Geometry: final body of the model. Coordinates: model frame, mm. Face numbers are marked on the shaded views. A direction names the side the tool comes from. Round coordinates to 2 decimals unless told otherwise and drop trailing zeros. Write each loop counter-clockwise with the first axis right and the second up, starting at its lowest first coordinate (ties: lowest second). Pieces come first, ordered by that corner, then holes. Notation, with made-up numbers: M 48,-34 L 74,-34 A20 cw 74,1 Z; hole C 14.5,78.5 d10. An arc over 180 degrees is marked long. Use one line per item in the form item = value. Start each with the question number.
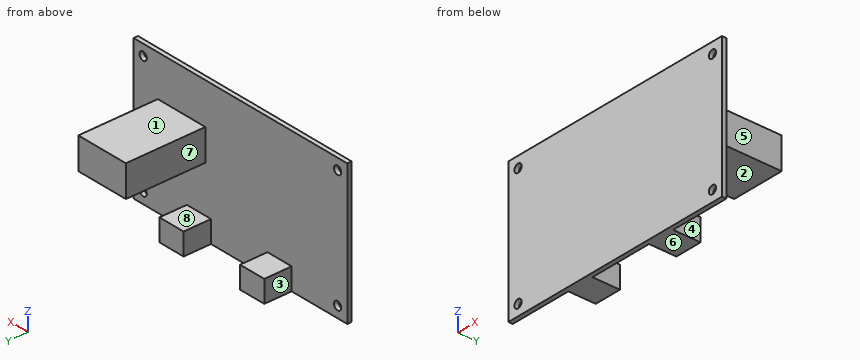
from build123d import *

# Parameters (mm, degrees)
ESQUISSE1_W        = 88.36
ESQUISSE1_H        = 51.38
ESQUISSE1_R        = 1.5
BOSS_EXTRU_2_DEPTH = 1.6
ESQUISSE3_W        = 10
ESQUISSE3_H        = 8
BOSS_EXTRU_3_DEPTH = 10
ESQUISSE4_W        = 19.65008467
ESQUISSE4_H        = 11.451158756
BOSS_EXTRU_4_DEPTH = 29


with BuildPart() as part:
    # Esquisse1 → Boss.-Extru.2 (new body)
    with BuildSketch(Plane(origin=(0, 0, 0), x_dir=(1, 0, 0), z_dir=(0, 1, 0))):
        with Locations((12.941904762, 5.88047619)):
            Rectangle(ESQUISSE1_W, ESQUISSE1_H)
        with Locations(Location((-27.238095238, -15.80952381, 0), (0, 0, 270))):
            Circle(ESQUISSE1_R, mode=Mode.SUBTRACT)
        with Locations(Location((53.171904762, -15.80952381, 0), (0, 0, 270))):
            Circle(ESQUISSE1_R, mode=Mode.SUBTRACT)
        with Locations(Location((53.171904762, 27.55047619, 0), (0, 0, 270))):
            Circle(ESQUISSE1_R, mode=Mode.SUBTRACT)
        with Locations(Location((-27.238095238, 27.55047619, 0), (0, 0, 270))):
            Circle(ESQUISSE1_R, mode=Mode.SUBTRACT)
    extrude(amount=BOSS_EXTRU_2_DEPTH)

    # Esquisse3 → Boss.-Extru.3 (add)
    with BuildSketch(Plane(origin=(0, 1.6, 0), x_dir=(1, 0, 0), z_dir=(0, 1, 0))):
        with Locations((30.121904762, 27.57047619)):
            Rectangle(ESQUISSE3_W, ESQUISSE3_H)
        with Locations((-3.238095238, 27.57047619)):
            Rectangle(ESQUISSE3_W, ESQUISSE3_H)
    extrude(amount=BOSS_EXTRU_3_DEPTH)

    # Esquisse4 → Boss.-Extru.4 (add)
    with BuildSketch(Plane(origin=(0, 1.6, 0), x_dir=(1, 0, 0), z_dir=(0, 1, 0))):
        with Locations((37.296862427, 0.916055568)):
            Rectangle(ESQUISSE4_W, ESQUISSE4_H)
    extrude(amount=BOSS_EXTRU_4_DEPTH)


solid = part.part
1. Section query B-B (x = 37.5). Return loops of the section in (y, z), then the cut area to 3 significant figures.
2. Set-up query: the marked faces 1, 2, 3, 4 and 5. Return all of +Z, -Z, +X, -X, +Y, -Y with unobstructed straight access to the full face (end or side cutting, diameter ignored); none if empty.
3. Pull-direction query (Z, two-part tool) for the marked faces 6, 7 and 8; classes: released by +Z, released by -Z, zero draft, split by the parting line, or undercut.
4. Section query A-A (y = 7). Return loops of the section in (x, z).
5. Ray query, probe 1 along Z at (x, y) = (29, 4.5); probe 2 along Y at (x, z) = (-16.5, 7); probe 3 along Z at (x, y) = (1.5, 8.5). Return the intervals inside material, ascending.
6. Contact query for flat-ended pins moving along their axis: pin 1 (1 mm diameter, centred on y = 22, z = 2.5, fed in from -X); pin 2 (4 mm diameter, centred on y = 4.5, z = -29, fed in from -X); pin 3 (5 mm diameter, centred on x = -27.24, z = 15.81, fed in from +Y). Output: stop coordinate, or through.
7. Section query D-D (y = 24). Return loops of the section in (x, z), then the cut area to 3 significant figures.
8. Section query C-C (z = -4). Return loops of the section in (x, y).
Checks:
q1.outline = M 0,-31.57 L 1.6,-31.57 L 1.6,-6.64 L 30.6,-6.64 L 30.6,4.81 L 1.6,4.81 L 1.6,19.81 L 0,19.81 Z
q1.area = 414 mm^2
q2.face_1 = +Z, +X, -X, +Y
q2.face_2 = +X, -X, +Y
q2.face_3 = +Z, -Z, -X, +Y
q2.face_4 = -Z, +X, +Y
q2.face_5 = +Z, -Z, +X, +Y
q3.face_6 = released by -Z
q3.face_7 = zero draft
q3.face_8 = undercut
q4.outline = M -8.24,-31.57 L 1.76,-31.57 L 1.76,-23.57 L -8.24,-23.57 Z; M 25.12,-31.57 L 35.12,-31.57 L 35.12,-23.57 L 25.12,-23.57 Z; M 27.47,-6.64 L 47.12,-6.64 L 47.12,4.81 L 27.47,4.81 Z
q5.probe_1 = -31.57 to -23.57, -6.64 to 4.81
q5.probe_2 = 0 to 1.6
q5.probe_3 = -31.57 to -23.57
q6.pin_1 = 27.47
q6.pin_2 = -8.24
q6.pin_3 = 1.6
q7.outline = M 27.47,-6.64 L 47.12,-6.64 L 47.12,4.81 L 27.47,4.81 Z
q7.area = 225 mm^2
q8.outline = M -31.24,0 L 57.12,0 L 57.12,1.6 L 47.12,1.6 L 47.12,30.6 L 27.47,30.6 L 27.47,1.6 L -31.24,1.6 Z
